The listing builds one solid part. Answer for the finished solid, in the listing's coordinates (mm). A direction names the side the tool comes from. Coordinates: 2 decimals unless noted, no trailing zeros. Order: outer loops, then holes, each group sorted by start corner. A loop starts at its lowest first (then second) coordinate and runs counter-clockwise, first axis right, second up. Notation, with made-up numbers: (26, 65.25) -> (41, 65.25) arc R27 ccw to (41, 96.25) -> close; hole circle Ø10 at (89, 46.5). An arc over 180 degrees is marked (long way). Write each question's results on one line, items separated by ' | '. Start each with the question number.
(1) Straight lines are drawn through the part: L1, parallel to Y at x = 74, z = 184; L2, parallel to Y at x = -77.5, z = 193.5; L3, parallel to Y at x = 1, z = 69.5. For each, find the intervals that lie inside material, in ascending order.
(2) The part is cut by section B-B, the plane z = 104. Give the vertices of the cut face in (x, y), then the cut area to 3 significant figures.
(3) Given pin 1 (6 mm diameter, centred on y = 7.5, z = 130.5, fed in from -X); pin 2 (5 mm diameter, centred on x = 73, z = 164.5, fed in from +Y); pin 3 (12 mm diameter, centred on x = 89, z = 200, fed in from -Y), each flat-ended and moving along its own axis, determine where each tip first touches the part or whether it passes through.
(4) Determine the mould class of faces 6 (the face through (-2, 22, 0)), 7 (the face through (-1.68, 27.395, 59.93)), 8 (the face through (-1, 0, 118)) for opening direction Y: +Y half, -Y half, draft (parallel to the pull), parting line (faces both ways), or undercut.
(5) A tool of negligible diameter and unlimited length cuts with its end or side. For faces 1 (the face through (92, 15, 118)), 2 (the face through (-2, 20, 121)), 3 (the face through (-69.79, 7.6, 118.32)), 4 (the face through (-120, 18, 118)), 5 (the face through (-2, 22, 240)), from which of +Z, -Z, +X, -X, +Y, -Y can it reach the whole face along a straight path? Write none if from no direction.
(6) The part is cut by section C-C, the plane x = 82. Give the vertices of the cut face in (y, z).
(7) The part is cut by section A-A, the plane y = 26. Give the vertices of the cut face in (x, z).
(8) The part is cut by section D-D, the plane y = 3.5. Give the vertices of the cut face in (x, z).
```python
from build123d import *

# Parameters (mm, degrees)
EXTRUDE_1_DEPTH     = 240
CUT_EXTRUDE_1_DEPTH = 241


with BuildPart() as part:
    # Эскиз1 → Бобышка-Вытянуть1 (new body)
    with BuildSketch(Plane.XY):
        Polygon((0, 0), (75, 0), (64.72, 15), (120, 15), (120, 35), (0, 35), (-120, 35), (-120, 15), (-64.72, 15), (-75, 0), align=None)
    extrude(amount=EXTRUDE_1_DEPTH)

    # Эскиз2 → Вырез-Вытянуть1 (cut, through all)
    with BuildSketch(Plane.ZY.offset(120)):
        Polygon((65, 35), (175, 35), (185, 20), (55, 20), align=None)
    extrude(amount=-CUT_EXTRUDE_1_DEPTH, mode=Mode.SUBTRACT)


solid = part.part
```
Established:
1) L1: y = 0 to 1.46, 15 to 20, 21.5 to 35 | L2: y = 15 to 35 | L3: y = 0 to 20
2) outline: (-120, 15) -> (-64.72, 15) -> (-75, 0) -> (75, 0) -> (64.72, 15) -> (120, 15) -> (120, 20) -> (-120, 20) -> close | area: 3,300 mm^2
3) pin 1: stops at x = -71.92 | pin 2: stops at y = 20 | pin 3: stops at y = 15
4) face 6: draft | face 7: undercut | face 8: -Y half
5) face 1: +Z, -Z, +X | face 2: +X, -X | face 3: +Z, -Z, -X | face 4: +Z, -Z, -X, +Y, -Y | face 5: +Z, +X, -X, +Y, -Y
6) outline: (15, 0) -> (35, 0) -> (35, 65) -> (20, 55) -> (20, 185) -> (35, 175) -> (35, 240) -> (15, 240) -> close
7) outline: (-120, 0) -> (120, 0) -> (120, 59) -> (-120, 59) -> close; (-120, 181) -> (120, 181) -> (120, 240) -> (-120, 240) -> close
8) outline: (-72.6, 0) -> (72.6, 0) -> (72.6, 240) -> (-72.6, 240) -> close
